from build123d import *

# Parameters (mm, degrees)
F0_W      = 50
F0_H      = 10
F1_DEPTH  = 4
F2_W      = 3
F2_H      = 10
F3_DEPTH  = 20
F4_R      = 4.99999
F5_R      = 2
F6_DEPTH  = 25
F7_R      = 3
F8_DEPTH  = 25
F9_R      = 1
F10_DEPTH = 46
F11_R     = 1
F12_DEPTH = 25


# Not quite as in the source:
# - a fillet or chamfer is up to 0.001 mm smaller than in the source, because OpenCascade refuses the exact size


with BuildPart() as f1:
    # F0 (on Top) → F1 (new body)
    with BuildSketch(Plane.XY):
        Rectangle(F0_W, F0_H)
    extrude(amount=F1_DEPTH)

    # F2 (on face) → F3 (join)
    with BuildSketch(Plane.XY.offset(4)):
        with Locations((23.5, 0)):
            Rectangle(F2_W, F2_H)
        with Locations((-23.5, 0)):
            Rectangle(F2_W, F2_H)
    extrude(amount=F3_DEPTH)

    # F4 (radius 5 in the source; OpenCascade refuses exactly that, so slightly less here)
    f4_edges = [f1.edges().sort_by_distance(p)[0] for p in [
        (-23.5, -5, 24),
        (-23.5, 5, 24),
        (23.5, -5, 24),
        (23.5, 5, 24),
    ]]
    fillet(f4_edges, radius=F4_R)

    # F5 (on face) → F6 (cut)
    with BuildSketch(Plane.YZ.offset(25)):
        with Locations((0, 19)):
            Circle(F5_R)
    extrude(amount=-F6_DEPTH, mode=Mode.SUBTRACT)

    # F7 (on face) → F8 (cut)
    with BuildSketch(Plane.YZ.offset(-22)):
        with Locations((0, 19)):
            Circle(F7_R)
    extrude(amount=-F8_DEPTH, mode=Mode.SUBTRACT)

    # F9 (on face) → F10 (join)
    with BuildSketch(Plane.YZ.offset(-22)):
        with Locations((-3, 13)):
            Circle(F9_R)
        with Locations((3, 13)):
            Circle(F9_R)
    extrude(amount=F10_DEPTH)

    # F11 (on face) → F12 (cut)
    with BuildSketch(Plane(origin=(22, 0, 0), x_dir=(0, -1, 0), z_dir=(-1, 0, 0))):
        with Locations((0, 11.84)):
            Circle(F11_R)
    extrude(amount=-F12_DEPTH, mode=Mode.SUBTRACT)


solid = f1.part
Work out the finished part from the listing and answer in its coordinate system (mm). A direction names the side the tool comes from. Give positions to 0.01 mm unless a question says otherwise; leave off trailing zeros. Write each loop counter-clockwise with the first axis right and the second up, starting at its lowest first coordinate (ties: lowest second). Pieces come first, ordered by that corner, then holes.
Q1. For a pull along X with two mould halves and no side action, classify faces 1 (the face through (-25, 0, 12)), 2 (the face through (24, 0, 21)), 3 (the face through (0, 3, 12)) as released by +X, released by -X, zero draft, split by the parting line, or undercut.
Answer:
face 1: released by -X
face 2: zero draft
face 3: undercut
Q2. The part is cut by section C-C on y = 0.5. Give the vertices of the cut face in (x, z), and give its area (3 significant figures).
Answer:
outline: (-25, 0) - (25, 0) - (25, 10.97) - (22, 10.97) - (22, 4) - (-22, 4) - (-22, 16.04) - (-25, 16.04) - close; (-25, 21.96) - (-22, 21.96) - (-22, 23.97) - (-25, 23.97) - close; (22, 12.71) - (25, 12.71) - (25, 17.06) - (22, 17.06) - close; (22, 20.94) - (25, 20.94) - (25, 23.97) - (22, 23.97) - close
area: 285 mm2
Q3. Straight lines are drawn through the part: L1, parallel to Z at x = 24.2, y = 0; L2, parallel to X at y = 2.75, z = 14.5; L3, parallel to Z at x = 4.5, y = -3. For each, find the intervals that lie inside material, in ascending order.
Answer:
L1: z = 0 to 10.84, 12.84 to 17, 21 to 24
L2: x = -25 to -22, 22 to 25
L3: z = 0 to 4, 12 to 14
Q4. The part is cut by section A-A on z = 9. Give the vertices of the cut face in (x, y).
Answer:
outline: (-25, -5) - (-22, -5) - (-22, 5) - (-25, 5) - close; (22, -5) - (25, -5) - (25, 5) - (22, 5) - close
Q5. Given pin 1 (1 mm diameter, centred on x = 9.5, y = -4, fed in from +Z); pin 2 (4 mm diameter, centred on x = -12, y = -2.5, fed in from +Z); pin 3 (4.5 mm diameter, centred on y = 0, z = 19, fed in from +X); pin 4 (12 mm diameter, centred on x = -1.5, z = 16.5, fed in from +Y), each flat-ended and moving along its own axis, determine where each tip first touches the part or whether it passes through.
Answer:
pin 1: stops at z = 13.87
pin 2: stops at z = 14
pin 3: stops at x = 25
pin 4: stops at y = 4
Q6. The part is cut by section B-B on x = -11. Give the vertices of the cut face in (y, z).
Answer:
outline: (-5, 0) - (5, 0) - (5, 4) - (-5, 4) - close; circle Ø2 at (-3, 13); circle Ø2 at (3, 13)
Q7. A tool of negligible diameter and unlimited length cuts with its end or side. For faces 4 (the face through (23.48, 0.13, 12.83)), 5 (the face through (0, 0, 4)), 6 (the face through (0, -3, 12)), 7 (the face through (-23, -3, 23)), 8 (the face through (-23.48, -0.65, 16.07)), from which of +Z, -Z, +X, -X, +Y, -Y can it reach the whole face along a straight path? Write none if from no direction.
Answer:
face 4: +X
face 5: +Y, -Y
face 6: none
face 7: +Z, +X, -X, -Y
face 8: -X
